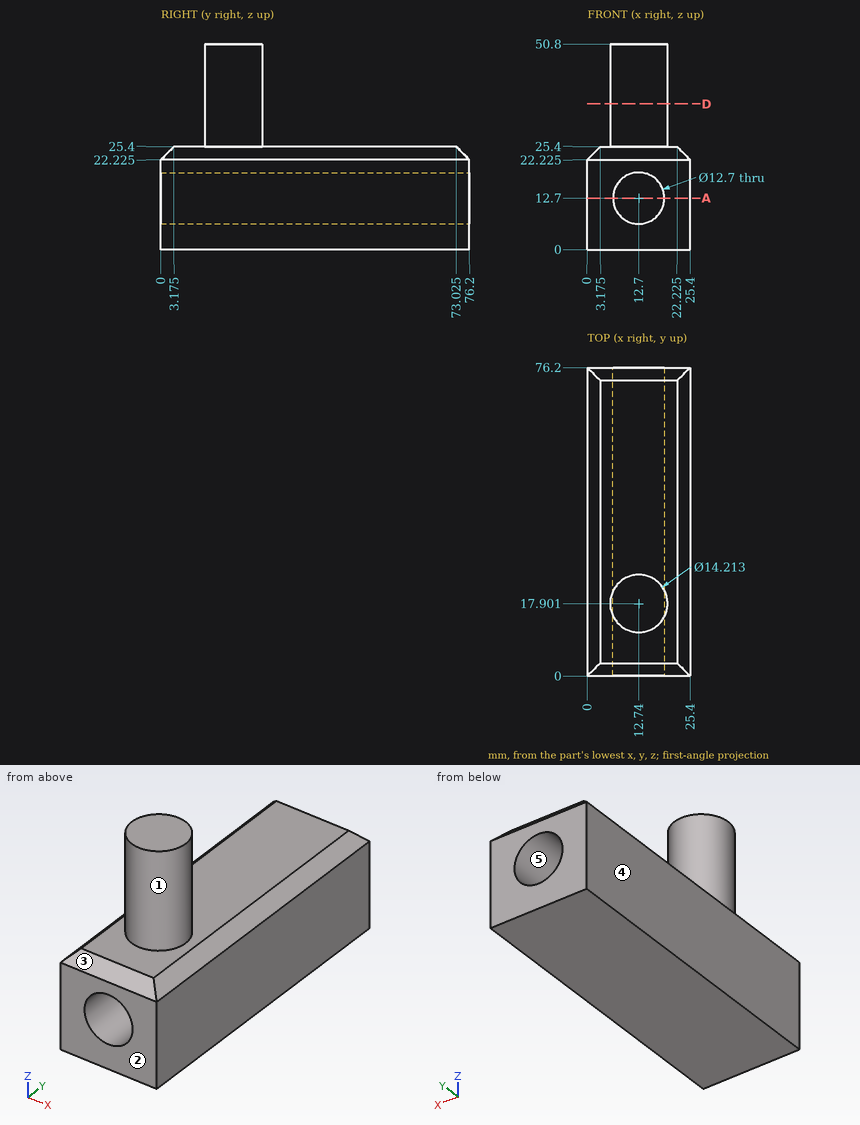
Answer from the drawing. Dimensions are ordinates in mm from the lowest x, y and z of the part. A direction names the side the tool comes from. Coordinates: 2 decimals unless noted, no trailing zeros. Write each loop counter-clockwise with the first axis right and the second up, starting at its lowest first coordinate (ties: lowest second). Pieces come first, ordered by that corner, then holes. Notation, with made-up numbers: M 68,50.25 L 117,50.25 A11 cw 117,63.25 Z; hole C 41,5.25 d8. An arc over 180 degrees is marked long. Use a Markdown table: item, result.
Q1. The part is cut by section A-A, the plane z = 12.7. Write down the section's boundary in (x, y).
Answer block:
| item | result |
|---|---|
| outline | M 0,0 L 6.35,0 L 6.35,76.2 L 0,76.2 Z; M 19.05,0 L 25.4,0 L 25.4,76.2 L 19.05,76.2 Z |
Q2. Which of the six approach directions +Z, -Z, +X, -X, +Y, -Y give full straight-line access (tool end or side, diameter ignored) to the marked faces 1 and 2?
Answer block:
| item | result |
|---|---|
| face 1 | +Z |
| face 2 | +Z, -Z, +X, -X, -Y |
Q3. Determine the mould class of the marked faces 3, 4 and 5 for opening direction Z: released by +Z, released by -Z, zero draft, split by the parting line, or undercut.
Answer block:
| item | result |
|---|---|
| face 3 | released by +Z |
| face 4 | zero draft |
| face 5 | undercut |
Q4. Each of these flat-tipped pins is pushed along its axis until it touches: pin 1 Ø8 at (x, y) = (18.5, 41.5) entering from +Z; pin 2 Ø1 at (x, z) = (15.5, 32) entering from -Y. Where does it stop, or does it pass through?
Answer block:
| item | result |
|---|---|
| pin 1 | stops at z = 25.4 |
| pin 2 | stops at y = 11.16 |
Q5. The part is cut by section D-D, the plane z = 36. Write down the section's boundary in (x, y).
Answer block:
| item | result |
|---|---|
| outline | C 12.74,17.9 d14.21 |
Q6. Straight lines are drawn through the part: L1, parallel to Z at x = 12.7, y = 49.5; L2, parallel to Z at x = 12.7, y = 19.5; L3, parallel to Z at x = 4.5, y = 72. For each, find the intervals that lie inside material, in ascending order. Write a range as [from, to].
Answer block:
| item | result |
|---|---|
| L1 | z = [0, 6.35], [19.05, 25.4] |
| L2 | z = [0, 6.35], [19.05, 50.8] |
| L3 | z = [0, 25.4] |
